```python
from build123d import *

# Parameters (mm, degrees)
F0_W     = 75
F0_H     = 75
F1_DEPTH = 20
F2_W     = 14
F2_H     = 14
F3_DEPTH = 12


with BuildPart() as f1:
    # F0 (on Top) → F1 (new body)
    with BuildSketch(Plane.XY):
        Rectangle(F0_W, F0_H)
    extrude(amount=F1_DEPTH)

    # F2 (on face) → F3 (cut)
    with BuildSketch(Plane.XY.offset(20)):
        Rectangle(F2_W, F2_H)
        with Locations((22.25, -22.25)):
            Rectangle(F2_W, F2_H)
        with Locations((22.25, 0)):
            Rectangle(F2_W, F2_H)
        with Locations((22.25, 22.25)):
            Rectangle(F2_W, F2_H)
        with Locations((0, 22.25)):
            Rectangle(F2_W, F2_H)
        with Locations((-22.25, 22.25)):
            Rectangle(F2_W, F2_H)
        with Locations((-22.25, 0)):
            Rectangle(F2_W, F2_H)
        with Locations((-22.25, -22.25)):
            Rectangle(F2_W, F2_H)
        with Locations((0, -22.25)):
            Rectangle(F2_W, F2_H)
    extrude(amount=-F3_DEPTH, mode=Mode.SUBTRACT)


solid = f1.part
```
The model under review builds one solid part; all positions refer to its coordinate system, in mm. A direction names the side the tool comes from. Round coordinates to 2 decimals unless told otherwise and drop trailing zeros. Loops run counter-clockwise (first coordinate to the right, second up) from the corner with the lowest first, then second, coordinate; pieces in that order, holes last. Notation, with made-up numbers: (7.25, -8.75) -> (53.25, -8.75) arc R30 cw to (53.25, 25.25) -> close; hole circle Ø1 at (64.5, 3.25). An arc over 180 degrees is marked (long way). Answer as a JSON object with one key per item and string values. Group by question number.
1) For line 1 (X direction, y = 18, z = 9.5); line 2 (Z direction, x = -28, y = -22), list the stretches that pass through material, from the lowest coordinate up. Write a range as [from, to].
2) Mouldability with a two-part tool opening along Y and no side actions: class faces 1 (the face through (-29.25, 22, 14)), 2 (the face through (-1, 1, 0)), 3 (the face through (-1, -37.5, 10)) as released by +Y, released by -Y, zero draft, split by the parting line, or undercut.
3) For faces 4 (the face through (-1, 9, 20)), 5 (the face through (-29.25, -22, 14)), list the 3-axis set-ups (+Z, -Z, +X, -X, +Y, -Y) from which the entire face can be reached by the end or side of a thin tool; tool diameter is ignored.
4) We need section C-C on z = 9. Give the number of separate pieces and of enclosed holes in the cut face, then the cut area to 3 significant figures.
5) For pin 1 Ø15.5 at (x, y) = (-22.5, 0.5) entering from +Z; pin 2 Ø7 at (x, y) = (-23, 21.5) entering from +Z, all flat-tipped, find the tip position at first contact; note any pin that passes through.
6) We need section A-A on x = 17. Write out the cut boundary in (y, z), then the cut area to 3 significant figures.
Result set:
{
 "1": {"line 1": "[-37.5, -29.25], [-15.25, -7], [7, 15.25], [29.25, 37.5]", "line 2": "[0, 8]"},
 "2": {"face 1": "undercut", "face 2": "zero draft", "face 3": "released by -Y"},
 "3": {"face 4": "+Z, +X, -X, +Y, -Y", "face 5": "+Z"},
 "4": {"separate pieces": "1", "enclosed holes": "9", "area": "3,860 mm²"},
 "5": {"pin 1": "z = 20", "pin 2": "z = 8"},
 "6": {"outline": "(-37.5, 0) -> (37.5, 0) -> (37.5, 20) -> (29.25, 20) -> (29.25, 8) -> (15.25, 8) -> (15.25, 20) -> (7, 20) -> (7, 8) -> (-7, 8) -> (-7, 20) -> (-15.25, 20) -> (-15.25, 8) -> (-29.25, 8) -> (-29.25, 20) -> (-37.5, 20) -> close", "area": "996 mm²"}
}
